Check sheet for the modelled part. Datum: model origin and axes. Units: mm. A direction names the side the tool comes from. Coordinates: 2 decimals unless noted, no trailing zeros. Loops run counter-clockwise (first coordinate to the right, second up) from the corner with the lowest first, then second, coordinate; pieces in that order, holes last.
Autodesk Inventor part; units mm, degrees
ref_plane "to_rring_1_XY" through (2.425, 0, 0) normal (1, 0, 0) x (0, 0, -1)
ref_plane "to_rring_1_YZ" through (2.425, 0, 0) normal (0, 0, -1) x (0, 1, 0)
ref_plane "to_rring_1_ZX" through (2.425, 0, 0) normal (0, 1, 0) x (1, 0, 0)
sketch "Sketch_1" plane through (0, 0, 0) normal (0, 1, 0) x (-1, 0, 0)
  line L0 (-131, 0) -> (0, 0)
  line L1 (0, 0) -> (0, -4.5)
  line L2 (0, -4.5) -> (-0.5, -5)
  line L3 (-0.5, -5) -> (-130.5, -5)
  line L4 (-130.5, -5) -> (-131, -4.5)
  line L5 (-131, -4.5) -> (-131, 0)
  line L6 (-131, 0) -> (0, 0)
revolve "Revolution1" add sketch "Sketch_1" angle 360 about axis through (131, 0, 0) along (1, 0, 0)
sketch "Sketch_27" plane through (0, 0, 0) normal (0, 0, 1) x (1, 0, 0)
  line L0 (131, 0) -> (-131, 0)
  line L1 (1.85, 9.6) -> (1.85, 4.8)
  line L2 (1.85, 4.8) -> (3, 4.8)
  line L3 (3, 4.8) -> (3, 9.6)
  line L4 (3, 9.6) -> (1.85, 9.6)
revolve "Revolution2" cut sketch "Sketch_27" angle 360 about axis through (131, 0, 0) along (1, 0, 0)
sketch "Sketch_39" plane through (0, 0, 0) normal (0, 0, 1) x (1, 0, 0)
  line L0 (131, 0) -> (-131, 0)
  line L1 (126, 9.6) -> (126, 4.8)
  line L2 (126, 4.8) -> (127.15, 4.8)
  line L3 (127.15, 4.8) -> (127.15, 9.6)
  line L4 (127.15, 9.6) -> (126, 9.6)
revolve "Revolution3" cut sketch "Sketch_39" angle 360 about axis through (131, 0, 0) along (1, 0, 0)
sketch "_____7" plane through (0, 0, 5) normal (0, 0, 1) x (1, 0, 0)
  arc A0 (6.5, 1.5) -> (6.5, -1.5) centre (6.5, 0) ccw
  line L0 (6.5, -1.5) -> (22.5, -1.5)
  arc A1 (22.5, -1.5) -> (22.5, 1.5) centre (22.5, 0) ccw
  line L1 (22.5, 1.5) -> (6.5, 1.5)
extrude "Extrusion1" cut sketch "_____7" against normal blind 1.8
sketch "_____10" plane through (0, 0, 5) normal (0, 0, 1) x (1, 0, 0)
  arc A0 (113, 1.5) -> (113, -1.5) centre (113, 0) ccw
  line L0 (113, -1.5) -> (121, -1.5)
  arc A1 (121, -1.5) -> (121, 1.5) centre (121, 0) ccw
  line L1 (121, 1.5) -> (113, 1.5)
extrude "Extrusion2" cut sketch "_____10" against normal blind 1.8
ref_plane "to_rring_1_XY" through (2.425, 0, 0) normal (1, 0, 0) x (0, 0, -1)
ref_plane "to_rring_1_YZ" through (2.425, 0, 0) normal (0, 0, -1) x (0, 1, 0)
ref_plane "to_rring_1_ZX" through (2.425, 0, 0) normal (0, 1, 0) x (1, 0, 0)
ref_plane "to_rring_2_XY" through (126.575, 0, 0) normal (1, 0, 0) x (0, 0, -1)
ref_plane "to_rring_2_YZ" through (126.575, 0, 0) normal (0, 0, -1) x (0, 1, 0)
ref_plane "to_rring_2_ZX" through (126.575, 0, 0) normal (0, 1, 0) x (1, 0, 0)
properties part number "NSFMKRRA10-131-F3-S5-KA5-A19-KB111.5-B11_s"
(1) Draft check along Y on faces 4 (the face through (0, 0, 0)), 5 (the face through (117, 0, 3.2)), 6 (the face through (2.43, 2.58, 4.05)). Enter one of: pulls with the +Y half, pulls with the -Y half, needs draft (parallel to the pull), parting line crosses it, or undercut.
(2) Set-up check for faces 1 (the face through (14, 0, 3.2)), 2 (the face through (126.58, 2.58, 4.05)), 3 (the face through (131, 0, 0)): record each of +Z, -Z, +X, -X, +Y, -Y from which the full face is reachable in a straight line by a thin tool's end or side.
(3) Section check B-B, the plane x = 28.5. Enter the section's corners in (y, z).
(4) Gauge pin test, flat ends, axial feed: P1, Ø0.9, axis at x = 13, y = 0, coming from the +Z side; P2, Ø6, axis at x = 38.5, z = 3.5, coming from the +Y side; P3, Ø1.7, axis at x = 15.5, z = 3.5, coming from the +Y side. Record the tip position at first contact, or that the pin passes through.
(5) Scan lines: line 1 along X through (y, z) = (-2, -4.5); line 2 along Y through (x, z) = (18.5, 0.25); line 3 along Z through (x, y) = (8, 0.5). Record each from-to range of solid material in increasing order.
Determined:
1. face 4: needs draft
1. face 5: undercut
1. face 6: parting line crosses it
2. face 1: +Z
2. face 2: none
2. face 3: +Z, -Z, +X, +Y, -Y
3. outline: circle Ø10 at (0, 0)
4. P1: stops at z = 3.2
4. P2: stops at y = 4.97
4. P3: stops at y = 4.24
5. line 1: x = 0.42 to 1.85, 3 to 126, 127.15 to 130.58
5. line 2: y = -4.99 to 4.99
5. line 3: z = -4.97 to 3.2
